Verification items for the finished model (mm, model axes). A direction names the side the tool comes from. Coordinates: 2 decimals unless noted, no trailing zeros. Order: outer loops, then holes, each group sorted by start corner. A loop starts at its lowest first (then second) coordinate and runs counter-clockwise, first axis right, second up. Notation, with made-up numbers: M 78.25,48 L 111.25,48 A32 ccw 111.25,86 Z; hole C 82,25.25 d9. An arc over 180 degrees is marked long. Answer as a JSON object with one key per item and string values. Group by question number.
(1) Access from +Z, -Z, +X, -X, +Y, -Y to the whole of each face (thin tool, end or side, straight path). Record for faces 5 (the face through (-11.328, 43.717, 27.552)), 6 (the face through (0, 25, 25)).
(2) Material ranges on line 1 (Z direction, x = -12.7, y = 46); line 2 (Y direction, x = -25.4, z = 14); line 3 (X direction, y = 41.75, z = 25.4), recorded low to high.
(3) Cross-section at B-B (z = 40). Enter the section's corners in (x, y) (3 decimals).
(4) Mould release check, pull along X, two halves, no side actions. Record for faces 1 (the face through (-26, 26, 50.8)), 2 (the face through (-12.642, 35.563, 25.84)), 3 (the face through (-50.8, 25, 25)), 4 (the face through (-24.702, 40.238, 25.044)): released by +X, released by -X, zero draft, split by the parting line, or undercut.
(5) Cross-section at A-A (x = -25.4). Enter the section's corners in (y, z).
from build123d import *

# Parameters (mm, degrees)
F0_W     = 50.8
F0_H     = 50.8
F1_DEPTH = 50.8
F3_D     = 10.71626
F5_D     = 5.1054
F5_DEPTH = 13.97
F5_TIP   = 1.5338169022


with BuildPart() as f1:
    # F0 (on Top) → F1 (new body)
    with BuildSketch(Plane.XY):
        with Locations((-25.4, 25.4)):
            Rectangle(F0_W, F0_H)
    extrude(amount=F1_DEPTH)

    # F3 (through all)
    with Locations(Plane.XY.offset(50.8)):
        with Locations((-25.4, 34.925)):
            Hole(F3_D / 2)

    # F5
    with Locations(Plane(origin=(0, 50.8, 0), x_dir=(-1, 0, 0), z_dir=(0, 1, 0))):
        with Locations((12.7, 25.4)):
            Hole(F5_D / 2, depth=F5_DEPTH)
            with Locations((0, 0, -(F5_DEPTH + F5_TIP / 2))):  # 118° drill point
                Cone(0, F5_D / 2, F5_TIP, mode=Mode.SUBTRACT)


solid = f1.part
Taken from the geometry:
{
 "1": {"face 5": "+Y", "face 6": "+Z, -Z, +X, +Y, -Y"},
 "2": {"line 1": "z = 0 to 22.85, 27.95 to 50.8", "line 2": "y = 0 to 29.57, 40.28 to 50.8", "line 3": "x = -50.8 to -15.25, -10.15 to 0"},
 "3": {"outline": "M -50.8,0 L 0,0 L 0,50.8 L -50.8,50.8 Z; hole C -25.4,34.925 d10.716"},
 "4": {"face 1": "zero draft", "face 2": "undercut", "face 3": "released by -X", "face 4": "undercut"},
 "5": {"outline": "M 0,0 L 29.57,0 L 29.57,50.8 L 0,50.8 Z; M 40.28,0 L 50.8,0 L 50.8,50.8 L 40.28,50.8 Z"}
}
